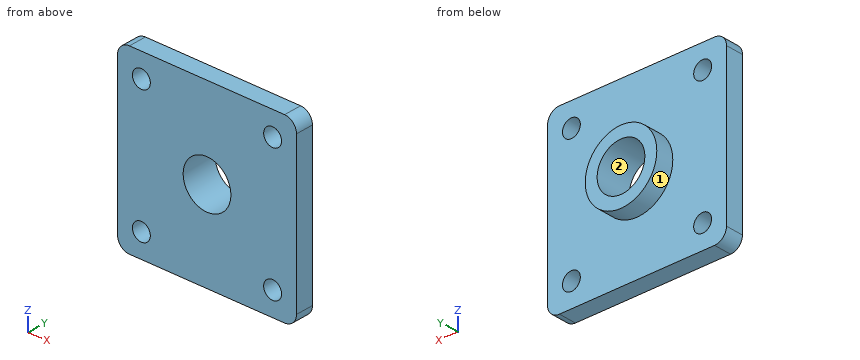
from build123d import *

# Parameters (mm, degrees)
SKETCH1_W          = 95.25
SKETCH1_H          = 95.25
EXTRUDE1_DEPTH     = 9.525
SKETCH2_R          = 19.05
EXTRUDE2_DEPTH     = 9.525
SKETCH3_R          = 12.7
CUT_EXTRUDE1_DEPTH = 20.05
FILLET1_R          = 6.35
CUT_EXTRUDE2_REACH = 11.525
SKETCH4_R          = 4.7625


with BuildPart() as part:
    # Sketch1 → Extrude1 (new body)
    with BuildSketch(Plane(origin=(0, 0, 0), x_dir=(1, 0, 0), z_dir=(0, 1, 0))):
        Rectangle(SKETCH1_W, SKETCH1_H)
    extrude(amount=EXTRUDE1_DEPTH)

    # Sketch2 → Extrude2 (add)
    with BuildSketch(Plane(origin=(0, 9.525, 0), x_dir=(-1, 0, 0), z_dir=(0, 1, 0))):
        Circle(SKETCH2_R)
    extrude(amount=EXTRUDE2_DEPTH)

    # Sketch3 → Cut-Extrude1 (cut, through all)
    with BuildSketch(Plane(origin=(0, 19.05, 0), x_dir=(-1, 0, 0), z_dir=(0, 1, 0))):
        Circle(SKETCH3_R)
    extrude(amount=-CUT_EXTRUDE1_DEPTH, mode=Mode.SUBTRACT)

    # Fillet1
    fillet1_edges = [part.edges().sort_by_distance(p)[0] for p in [
        (-47.625, 4.7625, -47.625),
        (47.625, 4.7625, -47.625),
        (47.625, 4.7625, 47.625),
        (-47.625, 4.7625, 47.625),
    ]]
    fillet(fillet1_edges, radius=FILLET1_R)

    # Sketch4 → Cut-Extrude2 (cut, up to next)
    with BuildSketch(Plane(origin=(0, 9.525, 0), x_dir=(-1, 0, 0), z_dir=(0, 1, 0)), mode=Mode.PRIVATE) as cut_extrude2_sk1:
        with Locations((-34.925, -34.925)):
            Circle(SKETCH4_R)
    cut_extrude2_tool1 = extrude(cut_extrude2_sk1.sketch, amount=-CUT_EXTRUDE2_REACH, mode=Mode.PRIVATE) & part.part
    add(cut_extrude2_tool1.solids().sort_by_distance((34.925, 9.525, -34.925))[0], mode=Mode.SUBTRACT)
    # Sketch4 → Cut-Extrude2 (cut, up to next)
    with BuildSketch(Plane(origin=(0, 9.525, 0), x_dir=(-1, 0, 0), z_dir=(0, 1, 0)), mode=Mode.PRIVATE) as cut_extrude2_sk2:
        with Locations((34.925, -34.925)):
            Circle(SKETCH4_R)
    cut_extrude2_tool2 = extrude(cut_extrude2_sk2.sketch, amount=-CUT_EXTRUDE2_REACH, mode=Mode.PRIVATE) & part.part
    add(cut_extrude2_tool2.solids().sort_by_distance((-34.925, 9.525, -34.925))[0], mode=Mode.SUBTRACT)
    # Sketch4 → Cut-Extrude2 (cut, up to next)
    with BuildSketch(Plane(origin=(0, 9.525, 0), x_dir=(-1, 0, 0), z_dir=(0, 1, 0)), mode=Mode.PRIVATE) as cut_extrude2_sk3:
        with Locations((34.925, 34.925)):
            Circle(SKETCH4_R)
    cut_extrude2_tool3 = extrude(cut_extrude2_sk3.sketch, amount=-CUT_EXTRUDE2_REACH, mode=Mode.PRIVATE) & part.part
    add(cut_extrude2_tool3.solids().sort_by_distance((-34.925, 9.525, 34.925))[0], mode=Mode.SUBTRACT)
    # Sketch4 → Cut-Extrude2 (cut, up to next)
    with BuildSketch(Plane(origin=(0, 9.525, 0), x_dir=(-1, 0, 0), z_dir=(0, 1, 0)), mode=Mode.PRIVATE) as cut_extrude2_sk4:
        with Locations((-34.925, 34.925)):
            Circle(SKETCH4_R)
    cut_extrude2_tool4 = extrude(cut_extrude2_sk4.sketch, amount=-CUT_EXTRUDE2_REACH, mode=Mode.PRIVATE) & part.part
    add(cut_extrude2_tool4.solids().sort_by_distance((34.925, 9.525, 34.925))[0], mode=Mode.SUBTRACT)


solid = part.part
Geometry check sheet. Reference: the model listing, model coordinates, mm. Face numbers are marked on the shaded views. A direction names the side the tool comes from. Give positions to 0.01 mm unless a question says otherwise; leave off trailing zeros. Loops run counter-clockwise (first coordinate to the right, second up) from the corner with the lowest first, then second, coordinate; pieces in that order, holes last.
(1) Section check C-C on z = 38. Record the cut outline in (x, y) (3 decimals).
From the geometry:
outline: (-47.625, 0) - (-38.562, 0) - (-38.562, 9.525) - (-47.625, 9.525) - close; (-31.288, 0) - (31.288, 0) - (31.288, 9.525) - (-31.288, 9.525) - close; (38.562, 0) - (47.625, 0) - (47.625, 9.525) - (38.562, 9.525) - close
(2) Depth check by flat-ended pin: pin 1 Ø11 at (x, z) = (-34.925, 34.925) entering from +Y (3 decimals). Enter the tip coordinate at first touch or a pass-through.
From the geometry:
pin 1: stops at y = 9.525
(3) Section check A-A on z = 0. Record the cut outline in (x, y) (3 decimals), then the cut area to 3 significant figures.
From the geometry:
outline: (-47.625, 0) - (-12.7, 0) - (-12.7, 19.05) - (-19.05, 19.05) - (-19.05, 9.525) - (-47.625, 9.525) - close; (12.7, 0) - (47.625, 0) - (47.625, 9.525) - (19.05, 9.525) - (19.05, 19.05) - (12.7, 19.05) - close
area: 786 mm2
(4) Section check B-B on x = 0. Record the cut outline in (y, z) (3 decimals), then the cut area to 3 significant figures.
From the geometry:
outline: (0, -47.625) - (9.525, -47.625) - (9.525, -19.05) - (19.05, -19.05) - (19.05, -12.7) - (0, -12.7) - close; (0, 12.7) - (19.05, 12.7) - (19.05, 19.05) - (9.525, 19.05) - (9.525, 47.625) - (0, 47.625) - close
area: 786 mm2
(5) Set-up check for the marked faces 1 and 2: record each of +Z, -Z, +X, -X, +Y, -Y from which the full face is reachable in a straight line by a thin tool's end or side.
From the geometry:
face 1: +Y
face 2: +Y, -Y
(6) Thickness scan on L1, parallel to Z at x = 0, y = 14.5; L2, parallel to X at y = 7, z = 36.5 (3 decimals); L3, parallel to Z at x = -34, y = 4 (3 decimals). Record the ranges inside material, lowest first.
From the geometry:
L1: z = -19.05 to -12.7, 12.7 to 19.05
L2: x = -47.625 to -39.42, -30.43 to 30.43, 39.42 to 47.625
L3: z = -47.625 to -39.597, -30.253 to 30.253, 39.597 to 47.625
(7) Section check D-D on y = 10.75. Record the cut outline in (x, z), then the cut area to 3 significant figures.
From the geometry:
outline: circle Ø38.1 at (0, 0); hole circle Ø25.4 at (0, 0)
area: 633 mm2
